For this review, take the finished solid that the model builds, in its own axes (mm). Face numbers are marked on the shaded views. A direction names the side the tool comes from. Round coordinates to 2 decimals unless told otherwise and drop trailing zeros. Order: outer loops, then holes, each group sorted by start corner. A loop starts at its lowest first (then second) coordinate and runs counter-clockwise, first axis right, second up. Notation, with made-up numbers: M -28.75,29.5 L 21.25,29.5 A14 ccw 21.25,34.5 Z; hole C -29,47.25 d4. An arc over 180 degrees is marked long. Use a Markdown table: item, result.
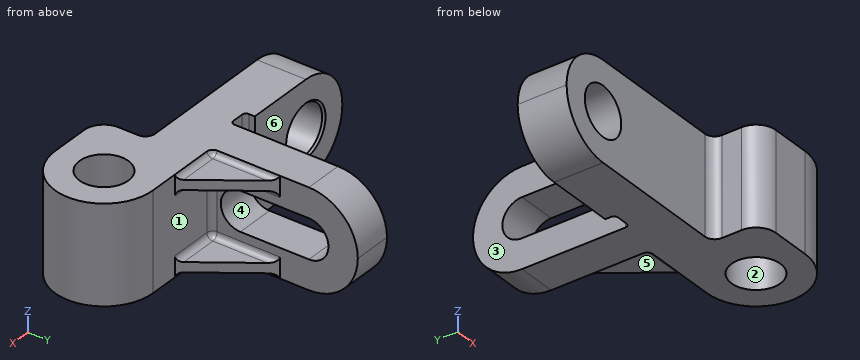
from build123d import *

# Parameters (mm, degrees)
ESBO_O1_R                              = 12.5
RESSALTO_EXTRUS_O1_DEPTH               = 25
FILETE1_R                              = 10
FILETE2_R                              = 5
FILETE3_R                              = 3
FILETE4_R                              = 2
FILETE5_R                              = 25
FURO_DE_DI_METRO_25_0_25_1_D           = 25
FURO_DE_DI_METRO_25_0_25_1_CSINK_D     = 27
FURO_DE_DI_METRO_25_0_25_1_CSINK_ANGLE = 90
CORTE_EXTRUS_O1_DEPTH                  = 50
NERVURA1_REACH                         = 191.868
ESBO_O6_WALL_W                         = 424.748377256
ESBO_O6_WALL_H                         = 5
FILETE6_R                              = 3


with BuildPart() as part:
    # Esboço1 → Ressalto-extrusão1 (new, symmetric)
    with BuildSketch(Plane.XY):
        with BuildLine():
            Line((0, 0), (0, 25))
            Line((0, 25), (60, 25))
            Line((60, 25), (60, 20))
            Line((60, 20), (70, 20))
            Line((70, 20), (70, 100))
            Line((70, 100), (90, 100))
            Line((90, 100), (90, 25.160806235))
            Line((90, 25.160806235), (130, 25.160806235))
            ThreePointArc((130, 25.160806235), (155, 0.160806235), (130, -24.839193765))
            Line((130, -24.839193765), (100, -24.839193765))
            Line((100, -24.839193765), (100, 0.160806235))
            Line((100, 0.160806235), (0, 0))
        make_face()
        with Locations((130, 0.160806235)):
            Circle(ESBO_O1_R, mode=Mode.SUBTRACT)
    extrude(amount=RESSALTO_EXTRUS_O1_DEPTH, both=True)

    # Filete1
    filete1_edges = [part.edges().sort_by_distance(p)[0] for p in [
        (100, -24.839193765, 0),
    ]]
    fillet(filete1_edges, radius=FILETE1_R)

    # Filete2
    filete2_edges = [part.edges().sort_by_distance(p)[0] for p in [
        (100, 0.160806235, 0),
    ]]
    fillet(filete2_edges, radius=FILETE2_R)

    # Filete3
    filete3_edges = [part.edges().sort_by_distance(p)[0] for p in [
        (90, 25.160806235, 0),
    ]]
    fillet(filete3_edges, radius=FILETE3_R)

    # Filete4
    filete4_edges = [part.edges().sort_by_distance(p)[0] for p in [
        (60, 20, 0),
        (70, 20, 0),
    ]]
    fillet(filete4_edges, radius=FILETE4_R)

    # Filete5
    filete5_edges = [part.edges().sort_by_distance(p)[0] for p in [
        (0, 12.5, -25),
        (0, 12.5, 25),
        (80, 100, 25),
        (80, 100, -25),
    ]]
    fillet(filete5_edges, radius=FILETE5_R - 0.0001)  # a hair under: the kernel refuses the full size

    # Furo de diâmetro Ø25.0 (25)1 (through all)
    with Locations(Plane(origin=(0, 25, 0), x_dir=(1, 0, 0), z_dir=(0, 1, 0))):
        with Locations((25, 0)):
            CounterSinkHole(FURO_DE_DI_METRO_25_0_25_1_D / 2, FURO_DE_DI_METRO_25_0_25_1_CSINK_D / 2, counter_sink_angle=FURO_DE_DI_METRO_25_0_25_1_CSINK_ANGLE)

    # Esboço5 → Corte-extrusão1 (cut)
    with BuildSketch(Plane.ZY.offset(-70)):
        with BuildLine():
            Line((10, 75), (10, 40))
            ThreePointArc((10, 40), (0, 30), (-10, 40))
            Line((-10, 40), (-10, 75))
            ThreePointArc((-10, 75), (0, 85), (10, 75))
        make_face()
    extrude(amount=-CORTE_EXTRUS_O1_DEPTH, mode=Mode.SUBTRACT)

    # Esboço6 wall → Nervura1 (add, up to next)
    with BuildSketch(Plane(origin=(102.5, 42.660806235, 20), x_dir=(0.581238193719, -0.813733471207, 0), z_dir=(0.813733471207, 0.581238193719, 0)), mode=Mode.PRIVATE) as nervura1_sk1:
        Rectangle(ESBO_O6_WALL_W, ESBO_O6_WALL_H)
    nervura1_tool1 = extrude(nervura1_sk1.sketch, amount=-NERVURA1_REACH, mode=Mode.PRIVATE) - part.part
    add(nervura1_tool1.solids().sort_by_distance((102.5, 42.660806235, 20))[0])

    # Filete6
    # the kernel refuses this fillet: 3 mm, written as the material it adds along each edge
    with BuildSketch(Plane(origin=(122.5, 25.160806235, 17.5), x_dir=(0, 0, -1), z_dir=(-1, 0, 0))) as filete6_piece_1_section:
        with BuildLine():
            CenterArc((FILETE6_R, -FILETE6_R), FILETE6_R, 90, 90)
            Line((0, -FILETE6_R), (0, 0))
            Line((0, 0), (FILETE6_R, 0))
        make_face()
    filete6_piece_1 = extrude(amount=29.5, mode=Mode.PRIVATE)
    filete6_piece_1 = split(filete6_piece_1, bisect_by=Plane(origin=(117.533783784, 21.613508937, 17.5), z_dir=(-0.8137334712068701, -0.5812381937189072, 0)), keep=Keep.TOP, mode=Mode.PRIVATE)
    add(filete6_piece_1)
    with BuildSketch(Plane(origin=(93, 28.160806235, 17.5), x_dir=(0, -1, 0), z_dir=(1, 0, 0))) as filete6_piece_2:
        with BuildLine():
            CenterArc((3 - FILETE6_R, FILETE6_R), FILETE6_R, 270, 90)
            Line((3, FILETE6_R), (3, 0))
            Line((3, 0), (3 - FILETE6_R, 0))
        make_face()
    revolve(axis=Axis((93, 28.160806235, 17.5), (0, 0, -1)), revolution_arc=90)
    with BuildSketch(Plane(origin=(90, 28.160806235, 17.5), x_dir=(0, 0, -1), z_dir=(0, 1, 0))) as filete6_piece_3_section:
        with BuildLine():
            CenterArc((FILETE6_R, -FILETE6_R), FILETE6_R, 90, 90)
            Line((0, -FILETE6_R), (0, 0))
            Line((0, 0), (FILETE6_R, 0))
        make_face()
    filete6_piece_3 = extrude(amount=39.5, mode=Mode.PRIVATE)
    filete6_piece_3 = split(filete6_piece_3, bisect_by=Plane(origin=(105.135135135, 38.971617046, 17.5), z_dir=(-0.8137334712068701, -0.5812381937189072, 0)), keep=Keep.TOP, mode=Mode.PRIVATE)
    add(filete6_piece_3)
    with BuildSketch(Plane(origin=(93, 25.160806235, 22.5), x_dir=(0, 0, 1), z_dir=(1, 0, 0))) as filete6_piece_4_section:
        with BuildLine():
            CenterArc((3, -2.958039892), FILETE6_R, 99.594068227, 80.405931773)
            Line((0, -2.958039892), (0, 0))
            Line((0, 0), (2.5, 0))
        make_face()
    filete6_piece_4 = extrude(amount=29.395099729, mode=Mode.PRIVATE)
    filete6_piece_4 = split(filete6_piece_4, bisect_by=Plane(origin=(107.567567568, 35.56621164, 22.5), z_dir=(-0.8137334712068701, -0.5812381937189072, 0)), keep=Keep.TOP, mode=Mode.PRIVATE)
    add(filete6_piece_4)
    with BuildSketch(Plane(origin=(93, 28.160806235, 22.5), x_dir=(0, -1, 0), z_dir=(1, 0, 0))) as filete6_piece_5:
        with BuildLine():
            CenterArc((0.041960108, -3), FILETE6_R, 9.594068227, 80.405931773)
            Line((0.041960108, 0), (3, 0))
            Line((3, 0), (3, -2.5))
        make_face()
    revolve(axis=Axis((93, 28.160806235, 22.5), (0, 0, -1)), revolution_arc=90)
    with BuildSketch(Plane(origin=(90, 67.555905964, 22.5), x_dir=(0, 0, 1), z_dir=(0, -1, 0))) as filete6_piece_6_section:
        with BuildLine():
            CenterArc((3, -2.958039892), FILETE6_R, 99.594068227, 80.405931773)
            Line((0, -2.958039892), (0, 0))
            Line((0, 0), (2.5, 0))
        make_face()
    filete6_piece_6 = extrude(amount=39.395099729, mode=Mode.PRIVATE)
    filete6_piece_6 = split(filete6_piece_6, bisect_by=Plane(origin=(86.502317696, 65.057561461, 22.5), z_dir=(-0.8137334712068701, -0.5812381937189072, 0)), keep=Keep.TOP, mode=Mode.PRIVATE)
    add(filete6_piece_6)

    # Espelhar1: read off the stored shape, not the designer's step
    # Espelhar1: part across plane


with BuildPart() as part_1:
    add(part.part)
    add(part.part.mirror(Plane.XY))


solid = part_1.part
Q1. Add section B-B (y = 49.5). Write out the cut boundary in (x, z).
Determined:
| item | result |
|---|---|
| outline | M 70,-25 L 90,-25 A3 cw 92.96,-22.5 L 97.61,-22.5 L 97.61,-17.5 L 93,-17.5 A3 cw 90,-14.5 L 90,-10 L 70,-10 Z; M 70,10 L 90,10 L 90,14.5 A3 cw 93,17.5 L 97.61,17.5 L 97.61,22.5 L 92.96,22.5 A3 cw 90,25 L 70,25 Z |
Q2. Wall thickness on line 1 along Z through (x, y) = (25, 11); line 2 along X through (y, z) = (7.5, 0); line 3 along X through (y, z) = (84.5, -17.5): over which ranges is each line inside the solid? List them lowest first. Write a range as [from, to].
Determined:
| item | result |
|---|---|
| line 1 | z = [-25, -12.5], [12.5, 25] |
| line 2 | x = [0, 12.5], [37.5, 119.88], [140.12, 153.9] |
| line 3 | x = [70, 90] |
Q3. Add section A-A (y = 3.5). Give the number of separate pieces and of enclosed holes in the cut face, then the cut area to 3 significant figures.
Determined:
| item | result |
|---|---|
| separate pieces | 2 |
| enclosed holes | 1 |
| area | 5,780 mm^2 |
Q4. Machinability: for the marked faces 4, 5 and 6, which of the approach directions +Z, -Z, +X, -X, +Y, -Y give a long, thin tool a straight path to every point of the face, cutting with its end or side? Answer none if there is none.
Determined:
| item | result |
|---|---|
| face 4 | +X, -X |
| face 5 | -Z, +X, +Y |
| face 6 | +Z, -Z, -X, +Y |
Q5. Clearance check with flat-ended pins moving along their axes: pin 1 (10 mm diameter, centred on x = 102, y = 43.5, fed in from -Z); pin 2 (11 mm diameter, centred on y = -8, z = 7.5, fed in from -X); pin 3 (10 mm diameter, centred on x = 103, y = 37, fed in from +Z). State where each tip first meets the part, or that it passes through.
Determined:
| item | result |
|---|---|
| pin 1 | stops at z = -22.5 |
| pin 2 | stops at x = 99.41 |
| pin 3 | stops at z = 22.5 |
Q6. Draft analysis for pull direction Y (two halves, no side actions). For the marked faces 1, 2 and 3, state which applies: pulls with the +Y half, pulls with the -Y half, needs draft (parallel to the pull), parting line crosses it, or undercut.
Determined:
| item | result |
|---|---|
| face 1 | pulls with the +Y half |
| face 2 | undercut |
| face 3 | needs draft |
